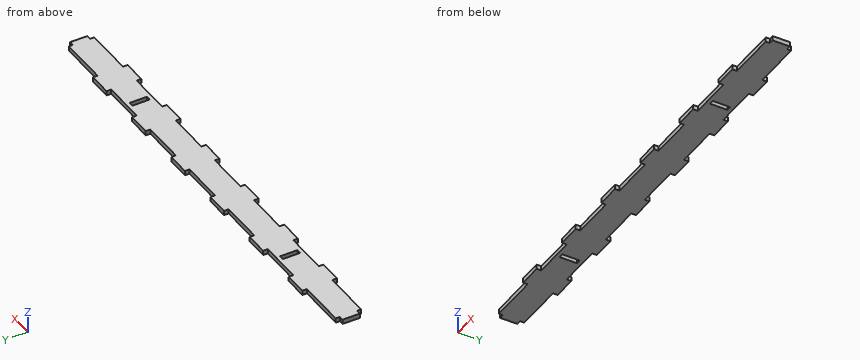
Autodesk Inventor part; units mm, degrees
ref_plane "YZ Plane" through (0, 0, 0) normal (1, 0, 0) x (0, 1, 0)
ref_plane "XZ Plane" through (0, 0, 0) normal (0, 1, 0) x (-1, 0, 0)
ref_plane "XY Plane" through (0, 0, 0) normal (0, 0, 1) x (1, 0, 0)
sketch "Sketch1" plane through (0, 0, 0) normal (0, 0, 1) x (1, 0, 0)
  line L0 (0, 6.16) -> (0, -6.16) construction
  line L1 (-109.76, 0) -> (109.76, 0) construction
  line L2 (78.4, -4.4) -> (-78.4, -4.4)
  line L3 (-78.4, -4.4) -> (-78.4, 4.4)
  line L4 (-78.4, 4.4) -> (78.4, 4.4)
  line L5 (78.4, 4.4) -> (78.4, -4.4)
  line L6 (78.4, -4.4) -> (-78.4, 4.4) construction
  line L7 (-78.4, -4.4) -> (78.4, 4.4) construction
  point P0 (0, 0)
  dimension "d0" = 156.8
  dimension "d1" = 8.8
extrude "Extrusion1" add sketch "Sketch1" along normal mid plane 1.6
sketch "Esquisse3" plane through (0, 0, 0.8) normal (0, 0, 1) x (1, 0, 0)
  line L0 (-78.4, -4.4) -> (78.4, -4.4) construction
  line L1 (78.4, -4.4) -> (78.4, 4.4) construction
  line L2 (78.4, 4.4) -> (-78.4, 4.4) construction
  line L3 (-78.4, 4.4) -> (-78.4, -4.4) construction
  line L4 (-112, 0) -> (112, 0) construction
  line L5 (0, 8.08) -> (0, -6.48) construction
  line L6 (-78.4, 3) -> (-80, 3)
  line L7 (-80, 3) -> (-80, -3)
  line L8 (-80, -3) -> (-78.4, -3)
  line L9 (-78.4, -3) -> (-78.4, 3)
  line L10 (78.4, 3) -> (80, 3)
  line L11 (80, 3) -> (80, -3)
  line L12 (80, -3) -> (78.4, -3)
  line L13 (78.4, -3) -> (78.4, 3)
  point P0 (0, 0)
  dimension "d15" = 1.6
  dimension "d16" = 6
extrude "Extrusion3" add sketch "Esquisse3" against normal blind 1.6
sketch "Esquisse4" plane through (0, 0, 0.8) normal (0, 0, 1) x (1, 0, 0)
  line L0 (80, 3) -> (80, -3) construction
  line L1 (80, -3) -> (78.4, -3) construction
  line L2 (78.4, -3) -> (78.4, -4.4) construction
  line L3 (78.4, -4.4) -> (-78.4, -4.4) construction
  line L4 (-78.4, -4.4) -> (-78.4, -3) construction
  line L5 (-78.4, -3) -> (-80, -3) construction
  line L6 (-80, -3) -> (-80, 3) construction
  line L7 (-80, 3) -> (-78.4, 3) construction
  line L8 (-78.4, 3) -> (-78.4, 4.4) construction
  line L9 (-78.4, 4.4) -> (78.4, 4.4) construction
  line L10 (78.4, 4.4) -> (78.4, 3) construction
  line L11 (78.4, 3) -> (80, 3) construction
  line L12 (-78.4, -4.4) -> (78.4, -4.4) construction
  line L13 (78.4, -4.4) -> (78.4, -3) construction
  line L14 (78.4, -3) -> (80, -3) construction
  line L15 (80, -3) -> (80, 3) construction
  line L16 (80, 3) -> (78.4, 3) construction
  line L17 (78.4, 3) -> (78.4, 4.4) construction
  line L18 (78.4, 4.4) -> (-78.4, 4.4) construction
  line L19 (-78.4, 4.4) -> (-78.4, 3) construction
  line L20 (-78.4, 3) -> (-80, 3) construction
  line L21 (-80, 3) -> (-80, -3) construction
  line L22 (-80, -3) -> (-78.4, -3) construction
  line L23 (-78.4, -3) -> (-78.4, -4.4) construction
  line L24 (0, 8.08) -> (0, -6.48) construction
  line L25 (-112, 0) -> (112, 0) construction
  line L26 (-61.5, 4.4) -> (-53.5, 4.4)
  line L27 (-53.5, 4.4) -> (-53.5, 6)
  line L28 (-53.5, 6) -> (-61.5, 6)
  line L29 (-61.5, 6) -> (-61.5, 4.4)
  line L30 (-30.5, 4.4) -> (-30.5, 6)
  line L31 (-38.5, 4.4) -> (-30.5, 4.4)
  line L32 (-30.5, 6) -> (-38.5, 6)
  line L33 (-38.5, 6) -> (-38.5, 4.4)
  line L34 (-7.5, 4.4) -> (-7.5, 6)
  line L35 (-15.5, 4.4) -> (-7.5, 4.4)
  line L36 (-7.5, 6) -> (-15.5, 6)
  line L37 (-15.5, 6) -> (-15.5, 4.4)
  line L38 (15.5, 4.4) -> (15.5, 6)
  line L39 (7.5, 4.4) -> (15.5, 4.4)
  line L40 (15.5, 6) -> (7.5, 6)
  line L41 (7.5, 6) -> (7.5, 4.4)
  line L42 (38.5, 4.4) -> (38.5, 6)
  line L43 (30.5, 4.4) -> (38.5, 4.4)
  line L44 (38.5, 6) -> (30.5, 6)
  line L45 (30.5, 6) -> (30.5, 4.4)
  line L46 (61.5, 4.4) -> (61.5, 6)
  line L47 (53.5, 4.4) -> (61.5, 4.4)
  line L48 (61.5, 6) -> (53.5, 6)
  line L49 (53.5, 6) -> (53.5, 4.4)
  point P0 (0, 0)
  dimension "d19" = 8
  dimension "d20" = 1.6
  dimension "d23" = 23
extrude "Extrusion4" add sketch "Esquisse4" against normal blind 1.6
mirror "Symétrie2" about plane through (0, 0, 0) normal (0, 1, 0) of "Extrusion4"
sketch "Esquisse5" plane through (0, 0, 0.8) normal (0, 0, 1) x (1, 0, 0)
  line L0 (45, -3) -> (43.4, -3)
  line L1 (43.4, -3) -> (43.4, 3)
  line L2 (43.4, 3) -> (45, 3)
  line L3 (45, 3) -> (45, -3)
  line L4 (-43.4, -3) -> (-45, -3)
  line L5 (-45, -3) -> (-45, 3)
  line L6 (-45, 3) -> (-43.4, 3)
  line L7 (-43.4, 3) -> (-43.4, -3)
  point P0 (0, 0)
extrude "Extrusion5" cut sketch "Esquisse5" against normal blind 1.6
properties part number "CaissonArriere" material "PVC-U"
Read the model definition and answer for the solid it produces. Units are mm, in the model's axes. Give positions to 0.01 mm unless a question says otherwise; leave off trailing zeros. Order: outer loops, then holes, each group sorted by start corner. A loop starts at its lowest first (then second) coordinate and runs counter-clockwise, first axis right, second up. Notation, with made-up numbers: (18, 84.5) -> (23, 84.5) arc R19 ccw to (23, 118.5) -> close; hole circle Ø11 at (-28.75, 29.25). An arc over 180 degrees is marked (long way). One line per item, written item: value. Start each with the question number.
(1) The part is cut by section B-B (z = 0.15). State how many separate pieces and enclosed holes the cut face has, and give its area (3 significant figures).
(2) Flat-ended cylindrical pins translate along their axes: P1, Ø0.5, axis at x = -79, z = 0.5, coming from the +Y side; P2, Ø0.5, axis at y = -5.5, z = 0, coming from the -X side; P3, Ø0.5, axis at x = 49.5, z = 0, coming from the -Y side. Find the tip coordinate at first contact, or state that the pin passes through.
(3) The part is cut by section C-C (x = 66). Determine the outline of the cut face in (y, z), and give its area (3 significant figures).
(4) Straight lines are drawn through the part: L1, parallel to X at y = 0.5, z = -0.7; L2, parallel to X at y = 4.75, z = -0.55; L3, parallel to Y at x = -63.5, z = 0.3. For each, find the intervals that lie inside material, in ascending order.
(5) The part is cut by section A-A (y = -0.5). Determine the outline of the cut face in (x, z), and give its area (3 significant figures).
Taken from the geometry:
1. separate pieces: 1
1. enclosed holes: 2
1. area: 1,530 mm^2
2. P1: y = 3
2. P2: x = -61.5
2. P3: y = -4.4
3. outline: (-4.4, -0.8) -> (4.4, -0.8) -> (4.4, 0.8) -> (-4.4, 0.8) -> close
3. area: 14.1 mm^2
4. L1: -80 to -45, -43.4 to 43.4, 45 to 80
4. L2: -61.5 to -53.5, -38.5 to -30.5, -15.5 to -7.5, 7.5 to 15.5, 30.5 to 38.5, 53.5 to 61.5
4. L3: -4.4 to 4.4
5. outline: (-80, -0.8) -> (-45, -0.8) -> (-45, 0.8) -> (-80, 0.8) -> close; (-43.4, -0.8) -> (43.4, -0.8) -> (43.4, 0.8) -> (-43.4, 0.8) -> close; (45, -0.8) -> (80, -0.8) -> (80, 0.8) -> (45, 0.8) -> close
5. area: 251 mm^2
